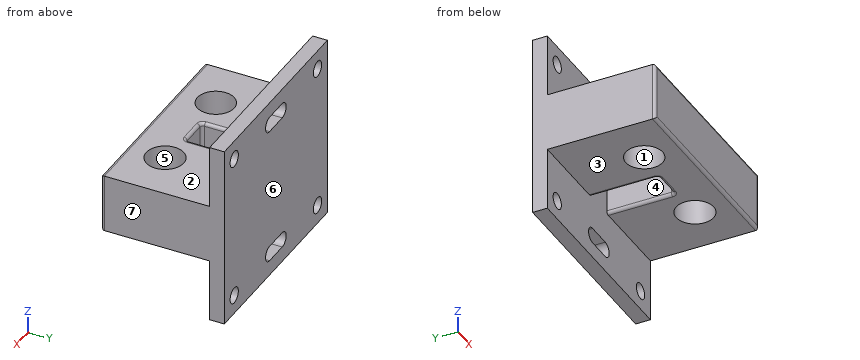
```python
from build123d import *

# Parameters (mm, degrees)
SKETCH1_W           = 65
SKETCH1_H           = 40
SKETCH1_R           = 6
SKETCH1_R_2         = 6.1
BOSS_EXTRUDE1_DEPTH = 19
SKETCH4_W           = 65
SKETCH4_H           = 14.8
BOSS_EXTRUDE2_DEPTH = 35
SKETCH6_W           = 10
SKETCH6_H           = 12
CUT_EXTRUDE1_DEPTH  = 45.5
CUT_EXTRUDE3_DEPTH  = 41
FILLET1_R           = 1
SKETCH9_W           = 65
SKETCH9_H           = 14.8
CUT_EXTRUDE4_DEPTH  = 5
SKETCH10_W          = 65
SKETCH10_H          = 14.8
CUT_EXTRUDE5_DEPTH  = 5
SKETCH11_R          = 2.6
CUT_EXTRUDE6_DEPTH  = 41
CUT_EXTRUDE7_DEPTH  = 10


with BuildPart() as part:
    # Sketch1 → Boss-Extrude1 (new body)
    with BuildSketch(Plane.XY):
        with Locations((14, 7.8)):
            Rectangle(SKETCH1_W, SKETCH1_H)
        with Locations((-2, 0)):
            Circle(SKETCH1_R, mode=Mode.SUBTRACT)
        with Locations((30, 0)):
            Circle(SKETCH1_R_2, mode=Mode.SUBTRACT)
    extrude(amount=-BOSS_EXTRUDE1_DEPTH)

    # Sketch4 → Boss-Extrude2 (add, symmetric)
    with BuildSketch(Plane.XY.offset(-9.5)):
        with Locations((14, 20.4)):
            Rectangle(SKETCH4_W, SKETCH4_H)
    extrude(amount=BOSS_EXTRUDE2_DEPTH, both=True)

    # Sketch6 → Cut-Extrude1 (cut, through all)
    with BuildSketch(Plane.XY):
        with Locations((14, 7)):
            Rectangle(SKETCH6_W, SKETCH6_H)
    extrude(amount=-CUT_EXTRUDE1_DEPTH, mode=Mode.SUBTRACT)

    # Sketch8 → Cut-Extrude3 (cut, through all)
    with BuildSketch(Plane(origin=(0, 27.8, 0), x_dir=(1, 0, 0), z_dir=(0, 1, 0))):
        with BuildLine():
            Line((18, 29.5), (10, 29.5))
            ThreePointArc((10, 29.5), (7.5, 32), (10, 34.5))
            Line((10, 34.5), (18, 34.5))
            ThreePointArc((18, 34.5), (20.5, 32), (18, 29.5))
        make_face()
        with BuildLine():
            Line((18, -10.5), (10, -10.5))
            ThreePointArc((10, -10.5), (7.5, -13), (10, -15.5))
            Line((10, -15.5), (18, -15.5))
            ThreePointArc((18, -15.5), (20.5, -13), (18, -10.5))
        make_face()
    extrude(amount=-CUT_EXTRUDE3_DEPTH, mode=Mode.SUBTRACT)

    # Fillet1
    fillet1_edges = [part.edges().sort_by_distance(p)[0] for p in [
        (14, 1, -19),
        (9, 7, -19),
        (19, 7, -19),
        (9, 1, -9.5),
        (19, 1, -9.5),
        (9, 7, 0),
        (14, 1, 0),
        (19, 7, 0),
        (14, -12.2, 0),
        (46.5, -12.2, -9.5),
        (-18.5, -12.2, -9.5),
        (14, -12.2, -19),
    ]]
    fillet(fillet1_edges, radius=FILLET1_R)

    # Sketch9 → Cut-Extrude4 (cut)
    with BuildSketch(Plane.XY.offset(25.5)):
        with Locations((14, 20.4)):
            Rectangle(SKETCH9_W, SKETCH9_H)
    extrude(amount=-CUT_EXTRUDE4_DEPTH, mode=Mode.SUBTRACT)

    # Sketch10 → Cut-Extrude5 (cut)
    with BuildSketch(Plane(origin=(0, 0, -44.5), x_dir=(-1, 0, 0), z_dir=(0, 0, -1))):
        with Locations((-14, 20.4)):
            Rectangle(SKETCH10_W, SKETCH10_H)
    extrude(amount=-CUT_EXTRUDE5_DEPTH, mode=Mode.SUBTRACT)

    # Sketch11 → Cut-Extrude6 (cut, through all)
    with BuildSketch(Plane(origin=(0, 27.8, 0), x_dir=(1, 0, 0), z_dir=(0, 1, 0))):
        with Locations((40.25, -14.25)):
            Circle(SKETCH11_R)
        with Locations((40.25, 33.25)):
            Circle(SKETCH11_R)
        with Locations((-12.25, 33.25)):
            Circle(SKETCH11_R)
        with Locations((-12.25, -14.25)):
            Circle(SKETCH11_R)
    extrude(amount=-CUT_EXTRUDE6_DEPTH, mode=Mode.SUBTRACT)

    # Sketch12 → Cut-Extrude7 (cut)
    with BuildSketch(Plane.XZ.offset(-13)):
        with BuildLine():
            Line((-18.5, -39.5), (46.5, -39.5))
            Line((46.5, -39.5), (46.5, -19))
            Line((46.5, -19), (20, -19))
            ThreePointArc((20, -19), (19.292893219, -18.707106781), (19, -18))
            Line((19, -18), (19, -1))
            ThreePointArc((19, -1), (19.292893219, -0.292893219), (20, 0))
            Line((20, 0), (46.5, 0))
            Line((46.5, 0), (46.5, 20.5))
            Line((46.5, 20.5), (-18.5, 20.5))
            Line((-18.5, 20.5), (-18.5, 0))
            Line((-18.5, 0), (8, 0))
            ThreePointArc((8, 0), (8.707106781, -0.292893219), (9, -1))
            Line((9, -1), (9, -18))
            ThreePointArc((9, -18), (8.707106781, -18.707106781), (8, -19))
            Line((8, -19), (-18.5, -19))
            Line((-18.5, -19), (-18.5, -39.5))
        make_face()
    extrude(amount=-CUT_EXTRUDE7_DEPTH, mode=Mode.SUBTRACT)


solid = part.part
```
Geometry check sheet. Reference: the model listing, model coordinates, mm. Face numbers are marked on the shaded views. A direction names the side the tool comes from. Round coordinates to 2 decimals unless told otherwise and drop trailing zeros. Loops run counter-clockwise (first coordinate to the right, second up) from the corner with the lowest first, then second, coordinate; pieces in that order, holes last. Notation, with made-up numbers: M 58.5,66.25 L 107.5,66.25 A23 ccw 107.5,80.25 Z; hole C 17,65 d8. An arc over 180 degrees is marked long. Return JSON: item names as keys, results as strings. Group by question number.
(1) Mould release check, pull along Y, two halves, no side actions. Record for the marked faces 4, 5, 6 and 7: pulls with the +Y half, pulls with the -Y half, needs draft (parallel to the pull), parting line crosses it, or undercut.
(2) Section check D-D, the plane z = -33.25. Enter the section's corners in (x, y), and give its area (3 significant figures).
(3) Scan lines: line 1 along Z through (x, y) = (-12.25, 25.2); line 2 along X through (y, z) = (25.9, -33.25); line 3 along X through (y, z) = (-4, -17.5). Record each from-to range of solid material in increasing order. Write a range as [from, to].
(4) Section check C-C, the plane x = -12.25. Enter the section's corners in (y, z), and give its area (3 significant figures).
(5) Section check B-B, the plane x = -2. Enter the section's corners in (y, z).
(6) Section check A-A, the plane y = 21. Enter the section's corners in (x, z).
(7) Go/stop test with flat-tipped pins: pin 1 (8.5 mm diameter, centred on x = -12.25, z = -33.25, fed in from -Y); pin 2 (17 mm diameter, centred on x = 1, y = 5, fed in from +Z); pin 3 (19.5 mm diameter, centred on x = 30, y = 0, fed in from -Z). Record where each tip stops, or that it passes through.
(8) Set-up check for the marked faces 1, 2 and 3: record each of +Z, -Z, +X, -X, +Y, -Y from which the full face is reachable in a straight line by a thin tool's end or side.
Data:
{
 "1": {"face 4": "undercut", "face 5": "undercut", "face 6": "pulls with the +Y half", "face 7": "needs draft"},
 "2": {"outline": "M -18.5,23 L -14.85,23 L -14.85,27.8 L -18.5,27.8 Z; M -9.65,23 L 7.83,23 L 7.83,27.8 L -9.65,27.8 Z; M 20.17,23 L 37.65,23 L 37.65,27.8 L 20.17,27.8 Z; M 42.85,23 L 46.5,23 L 46.5,27.8 L 42.85,27.8 Z", "area": "203 mm²"},
 "3": {"line 1": "[-39.5, -35.85], [-30.65, 11.65], [16.85, 20.5]", "line 2": "[-18.5, -14.85], [-9.65, 7.83], [20.17, 37.65], [42.85, 46.5]", "line 3": "[-18.5, -6.47], [2.47, 25.39], [34.61, 46.5]"},
 "4": {"outline": "M -12.2,-18 A1 ccw -11.2,-19 L 23,-19 L 23,-30.65 L 27.8,-30.65 L 27.8,11.65 L 23,11.65 L 23,0 L -11.2,0 A1 ccw -12.2,-1 Z; M 23,-39.5 L 27.8,-39.5 L 27.8,-35.85 L 23,-35.85 Z; M 23,16.85 L 27.8,16.85 L 27.8,20.5 L 23,20.5 Z", "area": "906 mm²"},
 "5": {"outline": "M -12.2,-18 A1 ccw -11.2,-19 L -6,-19 L -6,0 L -11.2,0 A1 ccw -12.2,-1 Z; M 6,-19 L 23,-19 L 23,-39.5 L 27.8,-39.5 L 27.8,20.5 L 23,20.5 L 23,0 L 6,0 Z"},
 "6": {"outline": "M -18.5,-19 L 8,-19 A1 ccw 9,-18 L 9,-1 A1 ccw 8,0 L -18.5,0 Z; M 19,-18 A1 ccw 20,-19 L 46.5,-19 L 46.5,0 L 20,0 A1 ccw 19,-1 Z"},
 "7": {"pin 1": "y = 23", "pin 2": "z = 0", "pin 3": "z = -19"},
 "8": {"face 1": "+Z, -Z", "face 2": "+Z, +X, -X, -Y", "face 3": "-Z, +X, -X, -Y"}
}
